from build123d import *

# Parameters (mm, degrees)
BOSS_EXTRUDE1_DEPTH = 2.5
BOSS_EXTRUDE2_DEPTH = 2.5
FILLET1_R           = 3


with BuildPart() as part:
    # Sketch1 → Boss-Extrude1 (new body)
    with BuildSketch(Plane.XY):
        with BuildLine():
            ThreePointArc((-36.498211921, -0.894837407), (-30.682272217, -2.600735992), (-24.91598031, -4.467584206))
            ThreePointArc((-24.91598031, -4.467584206), (-23.230561506, -3.577090815), (-21.328447916, -3.701906342))
            ThreePointArc((-21.328447916, -3.701906342), (-53.283170108, 5.003711479), (-86.182644365, 8.813783084))
            ThreePointArc((-86.182644365, 8.813783084), (-89.819650793, 5.456375715), (-86.462243424, 1.819369287))
            ThreePointArc((-86.462243424, 1.819369287), (-54.60957062, -1.869472767), (-23.671589589, -10.298093658))
            ThreePointArc((-23.671589589, -10.298093658), (-25.210339365, -9.214534302), (-25.965452096, -7.490684972))
            ThreePointArc((-25.965452096, -7.490684972), (-31.636424249, -5.655196046), (-37.356120498, -3.977692071))
            ThreePointArc((-37.356120498, -3.977692071), (-61.648333057, 1.290252949), (-86.386352251, 3.717853032))
            ThreePointArc((-86.386352251, 3.717853032), (-87.921167048, 5.380484542), (-86.258535538, 6.915299339))
            ThreePointArc((-86.258535538, 6.915299339), (-61.152151238, 4.451550721), (-36.498211921, -0.894837407))
        make_face()
        with BuildLine():
            ThreePointArc((-21.964443513, -5.492300042), (-21.192937962, -6.077210854), (-20.900018752, -7))
            ThreePointArc((-20.900018752, -7), (-21.577229606, -8.30708079), (-23.035593992, -8.507699958))
            ThreePointArc((-23.035593992, -8.507699958), (-24.498688375, -7.993907076), (-25.965452096, -7.490684972))
            ThreePointArc((-25.965452096, -7.490684972), (-25.210339365, -9.214534302), (-23.671589589, -10.298093658))
            ThreePointArc((-23.671589589, -10.298093658), (-20.481417495, -9.859239228), (-19.000018752, -7))
            ThreePointArc((-19.000018752, -7), (-19.640779524, -4.981398743), (-21.328447916, -3.701906342))
            ThreePointArc((-21.328447916, -3.701906342), (-23.230561506, -3.577090815), (-24.91598031, -4.467584206))
            ThreePointArc((-24.91598031, -4.467584206), (-23.438376962, -4.974656833), (-21.964443513, -5.492300042))
        make_face()
        with BuildLine():
            ThreePointArc((-23.035593992, -8.507699958), (-24.00771871, -6.46442476), (-21.964443513, -5.492300042))
            ThreePointArc((-21.964443513, -5.492300042), (-23.438376962, -4.974656833), (-24.91598031, -4.467584206))
            ThreePointArc((-24.91598031, -4.467584206), (-25.806449767, -5.852169897), (-25.965452096, -7.490684972))
            ThreePointArc((-25.965452096, -7.490684972), (-24.498688375, -7.993907076), (-23.035593992, -8.507699958))
        make_face()
        with BuildLine():
            ThreePointArc((-25.965452096, -7.490684972), (-25.806449767, -5.852169897), (-24.91598031, -4.467584206))
            ThreePointArc((-24.91598031, -4.467584206), (-30.682272217, -2.600735992), (-36.498211921, -0.894837407))
            ThreePointArc((-36.498211921, -0.894837407), (-35.385738878, -2.865219027), (-37.356120498, -3.977692071))
            ThreePointArc((-37.356120498, -3.977692071), (-31.636424249, -5.655196046), (-25.965452096, -7.490684972))
        make_face()
    extrude(amount=BOSS_EXTRUDE1_DEPTH)

    # Sketch2 → Boss-Extrude2 (add)
    with BuildSketch(Plane(origin=(0, 0, 0), x_dir=(-1, 0, 0), z_dir=(0, 0, -1))):
        with BuildLine():
            ThreePointArc((53.283170108, 5.003711479), (36.704107241, 2.974392367), (20.240739247, 0.156418643))
            ThreePointArc((20.240739247, 0.156418643), (18.734449346, -3.884474615), (19.201925094, -8.171570836))
            ThreePointArc((19.201925094, -8.171570836), (19.339488679, -5.496321293), (21.328447916, -3.701906342))
            ThreePointArc((21.328447916, -3.701906342), (37.141755573, 1.253074886), (53.283170108, 5.003711479))
        make_face()
    extrude(amount=-BOSS_EXTRUDE2_DEPTH)

    # Fillet1
    # the kernel refuses this fillet: 3 mm, written as the material it adds along each edge
    with BuildSketch(Plane(origin=(-53.283170108, 5.003711479, 0), x_dir=(-0.9819426110261866, 0.1891790386144179, 0), z_dir=(0, 0, 1))) as fillet1_piece_1:
        with BuildLine():
            CenterArc((0.138392848, -2.999999854), FILLET1_R, 90.017899156, 5.253257813)
            ThreePointArc((-0.137215119, -0.012686638), (-0.068606935, -0.006350072), (0, 0))
            ThreePointArc((0, 0), (0.068727825, -1.0735e-05), (0.13745565, 0))
        make_face()
    extrude(amount=2.5)
    # the kernel refuses this fillet: 3 mm, written as the material it takes off along each edge
    with BuildSketch(Plane(origin=(-20.240739247, 0.156418643, -4.239797149), x_dir=(0.4782853989003676, -0.8782044620694638, 0), z_dir=(0, 0, 1))) as fillet1_2_piece_1:
        with BuildLine():
            CenterArc((1.423846315, -2.987637282), FILLET1_R, 84.796647689, 55.779400765)
            ThreePointArc((-0.893558187, -1.082476824), (-0.447321739, -0.540790471), (0, 0))
            ThreePointArc((0, 0), (0.84795943, 0.03853047), (1.69591886, 0))
        make_face()
    extrude(amount=10.979594298, mode=Mode.SUBTRACT)


solid = part.part
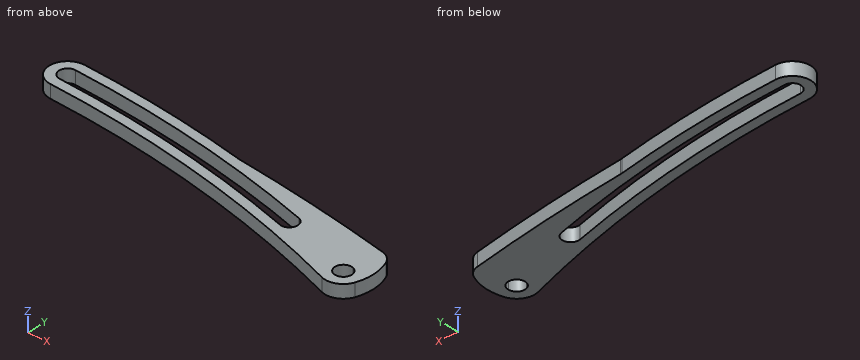
Work out the finished part from the listing and answer in its coordinate system (mm). Round coordinates to 2 decimals unless told otherwise and drop trailing zeros. Write each loop counter-clockwise with the first axis right and the second up, starting at its lowest first coordinate (ties: lowest second). Pieces come first, ordered by that corner, then holes. Notation, with made-up numbers: (34, 17.25) -> (40, 17.25) arc R22 cw to (40, 45.25) -> close; hole circle Ø7 at (74, 47.25). An arc over 180 degrees is marked (long way). Answer as CSV lines item,"result". Start each with the question number.
(1) The part is cut by section A-A, the plane z = 1.55. Give the vertices of the cut face in (x, y), then the cut area to 3 significant figures.
(2) Each of these flat-tipped pins is pushed along its axis until it touches: pin 1 (1 mm diameter, centred on x = -39, z = 1.5, fed in from -Y); pin 2 (10 mm diameter, centred on x = -46.5, y = -3, fed in from -Z); pin 3 (8 mm diameter, centred on x = -68.5, y = -5, fed in from -Z). Where does it stop, or does it pass through?
(3) The part is cut by section C-C, the plane x = -55. Give the vertices of the cut face in (y, z).
(4) The part is cut by section B-B, the plane y = 6.25. Give the vertices of the cut face in (x, z), then the cut area to 3 significant figures.
(5) Find the intervals of material crossed by probe 1 along Y at (x, z) = (-72.5, 1.6); probe 2 along Y at (x, z) = (-49, 1.2); probe 3 along Y at (x, z) = (-27.5, 0.75), in increasing order.
Output values:
1,outline,"(-86.46, 1.82) arc R213 cw to (-23.67, -10.3) arc R3.5 ccw to (-19.2, -8.17) arc R9.35 ccw to (-19.43, -1.33) arc R3 ccw to (-21.62, 0.42) arc R350 ccw to (-53.15, 4.99) arc R3 cw to (-53.42, 5.03) arc R220 ccw to (-86.18, 8.81) arc R3.5 ccw to start; hole (-86.39, 3.72) arc R214.9 cw to (-37.36, -3.98) arc R1.6 ccw to (-36.5, -0.89) arc R218.1 ccw to (-86.26, 6.92) arc R1.6 ccw to start; hole circle Ø3.2 at (-22.5, -7)"
1,area,"389 mm²"
2,pin 1,"stops at y = -5.63"
2,pin 2,"stops at z = 0"
2,pin 3,"passes through"
3,outline,"(-1.79, 0) -> (0.14, 0) -> (0.14, 2.5) -> (-1.79, 2.5) -> close; (3.4, 0) -> (5.33, 0) -> (5.33, 2.5) -> (3.4, 2.5) -> close"
4,outline,"(-89.7, 0) -> (-87.62, 0) -> (-87.62, 2.5) -> (-89.7, 2.5) -> close; (-75.85, 0) -> (-60.36, 0) -> (-60.36, 2.5) -> (-75.85, 2.5) -> close"
4,area,"43.9 mm²"
5,probe 1,"y = 0.8 to 2.71, 5.93 to 7.84"
5,probe 2,"y = -3.03 to -1.09, 2.19 to 4.56"
5,probe 3,"y = -8.98 to 1.5"
